Can you work these out from the model? Positions are in its coordinate system, mm. Give positions to 0.01 mm unless a question says otherwise; leave off trailing zeros. Loops run counter-clockwise (first coordinate to the right, second up) from the corner with the lowest first, then second, coordinate; pieces in that order, holes last. Notation, with made-up numbers: M 38,-20 L 85,-20 A21 cw 85,9 Z; hole C -22.5,58 d4. An arc over 180 degrees is marked long. Use CSV: the item, a comma, the result in double quotes.
from build123d import *

# Parameters (mm, degrees)
BOSS_EXTRUDE1_DEPTH      = 1
FILLET1_R                = 5
M5_CLEARANCE_HOLE1_D     = 5.8
M5_CLEARANCE_HOLE1_DEPTH = 5
M5_CLEARANCE_HOLE1_TIP   = 1.742495795
M3_CLEARANCE_HOLE1_D     = 3.6
CUT_EXTRUDE1_DEPTH       = 330.362644314
SKETCH10_R               = 2.1
CUT_EXTRUDE2_DEPTH       = 330.362644314


with BuildPart() as part:
    # Sketch1 → Boss-Extrude1 (new body)
    with BuildSketch(Plane(origin=(0, 0, 0), x_dir=(1, 0, 0), z_dir=(0, 1, 0))):
        Polygon((62.353829072, 0), (187.061487217, 0), (249.41531629, 108), (187.061487217, 216), (62.353829072, 216), (0, 108), align=None)
    extrude(amount=BOSS_EXTRUDE1_DEPTH)

    # Fillet1
    fillet1_edges = [part.edges().sort_by_distance(p)[0] for p in [
        (0, 0.5, -108),
        (62.353829072, 0.5, -216),
        (187.061487217, 0.5, -216),
        (249.41531629, 0.5, -108),
        (187.061487217, 0.5, 0),
        (62.353829072, 0.5, 0),
    ]]
    fillet(fillet1_edges, radius=FILLET1_R)

    # M5 Clearance Hole1
    with Locations(Plane(origin=(0, 1, 0), x_dir=(1, 0, 0), z_dir=(0, 1, 0))):
        with Locations((174.707658145, 146.57), (194.707658145, 146.57), (194.707658145, 196.57), (174.707658145, 196.57)):
            Hole(M5_CLEARANCE_HOLE1_D / 2, depth=M5_CLEARANCE_HOLE1_DEPTH)
            with Locations((0, 0, -(M5_CLEARANCE_HOLE1_DEPTH + M5_CLEARANCE_HOLE1_TIP / 2))):  # 118° drill point
                Cone(0, M5_CLEARANCE_HOLE1_D / 2, M5_CLEARANCE_HOLE1_TIP, mode=Mode.SUBTRACT)

    # M3 Clearance Hole1 (through all)
    with Locations(Plane(origin=(0, 1, 0), x_dir=(1, 0, 0), z_dir=(0, 1, 0))):
        with Locations((4.707658145, 108), (64.707658145, 211.923048454), (244.707658145, 108), (184.707658145, 4.076951546), (64.707658145, 4.076951546)):
            Hole(M3_CLEARANCE_HOLE1_D / 2)

    # Sketch9 → Cut-Extrude1 (cut, through all)
    with BuildSketch(Plane(origin=(0, 1, 0), x_dir=(1, 0, 0), z_dir=(0, 1, 0))):
        Polygon((195.835312633, 199.241777565), (196.511466747, 199.632155324), (198.261466747, 196.601066411), (197.585312633, 196.210688651), align=None)
    extrude(amount=-CUT_EXTRUDE1_DEPTH, mode=Mode.SUBTRACT)

    # Sketch10 → Cut-Extrude2 (cut, through all)
    with BuildSketch(Plane(origin=(0, 1, 0), x_dir=(1, 0, 0), z_dir=(0, 1, 0))):
        with Locations(Location((64.707658145, 21.923048454, 0), (0, 0, 270))):
            Circle(SKETCH10_R)
        with Locations(Location((214.707658145, 141.57, 0), (0, 0, 270))):
            Circle(SKETCH10_R)
        with Locations(Location((214.707658145, 121.57, 0), (0, 0, 270))):
            Circle(SKETCH10_R)
        with Locations(Location((214.707658145, 101.57, 0), (0, 0, 270))):
            Circle(SKETCH10_R)
        with Locations(Location((214.707658145, 81.57, 0), (0, 0, 270))):
            Circle(SKETCH10_R)
        with Locations(Location((234.707658145, 121.57, 0), (0, 0, 270))):
            Circle(SKETCH10_R)
    extrude(amount=-CUT_EXTRUDE2_DEPTH, mode=Mode.SUBTRACT)


solid = part.part
Q1. I want a section at A-A, the plane z = -146.57. Please give me the cut outline in (x, y).
Model answer:
outline,"M 22.27,0 L 171.81,0 L 171.81,1 L 22.27,1 Z; M 177.61,0 L 191.81,0 L 191.81,1 L 177.61,1 Z; M 197.61,0 L 227.15,0 L 227.15,1 L 197.61,1 Z"
Q2. I want a section at C-C, the plane x = 22.5. Please give me the cut outline in (y, z), then the cut area to 3 significant figures.
Model answer:
outline,"M 0,-146.97 L 1,-146.97 L 1,-69.03 L 0,-69.03 Z"
area,"77.9 mm2"
Q3. I want a section at B-B, the plane y = 0.6. State how many separate pieces and enclosed holes the cut face has, then the cut area to 3 significant figures.
Model answer:
separate pieces,"1"
enclosed holes,"14"
area,"40,200 mm2"
Q4. If we mould it in two halves opening along X, with no side actions, what happens to faces 1 (the flat face through (217.822, 0.493, -53.279)), 2 (the cylindrical face through (193.149, 0.493, -149.015)), 3 (the flat face through (123, 1, -110))? For each: released by +X, released by -X, zero draft, split by the parting line, or undercut.
Model answer:
face 1,"released by +X"
face 2,"undercut"
face 3,"zero draft"
Q5. Please list where these lines run through material, in increasing order: L1, parallel to X at y = 0.6, z = -121.57; L2, parallel to Z at x = 173, y = 0.8; L3, parallel to X at y = 0.6, z = -143.5. Write a range as from..to.
Model answer:
L1,"7.83..212.61, 216.81..232.61, 236.81..241.58"
L2,"-216..-198.91, -194.23..-148.91, -144.23..0"
L3,"20.5..213.88, 215.54..228.92"
Q6. I'm going to push a flat-ended pin straight in: P1, Ø3, axis at x = 184.71, z = -4.08, coming from the +Y side. Where does the tip first touch, or does it pass through?
Model answer:
P1,"through"
